The listing builds one solid part. Answer for the finished solid, in the listing's coordinates (mm). A direction names the side the tool comes from. Give positions to 0.01 mm unless a question says otherwise; leave off trailing zeros. Write each loop counter-clockwise with the first axis right and the second up, starting at its lowest first coordinate (ties: lowest second). Pieces come first, ordered by that corner, then holes. Notation, with made-up numbers: (2, -36) -> (36, -36) arc R21 cw to (36, -20) -> close; hole circle Ø6 at (9, 80.5). An arc over 180 degrees is marked (long way). Put each result on its own line as item: value. Start each with the question number.
1) A cutting plane is placed at B-B (y = 9.5). Write down the section's boundary in (x, z).
2) Find the intervals of material crossed by line 1 along X through (y, z) = (-8.75, 1.85); line 2 along X through (y, z) = (-0.75, 2.45); line 3 along Y through (x, z) = (12.5, 2.5), in increasing order. Write a range as from..to.
3) For a pull along X with two mould halves and no side action, classify faces 6 (the cylindrical face through (25.7, 0.5, 1.5)), 7 (the flat face through (20, -13.25, 1)), 8 (the flat face through (-36.5, 9, 1)) as released by +X, released by -X, zero draft, split by the parting line, or undercut.
4) Flat-ended cylindrical pins translate along their axes: pin 1 Ø2 at (y, z) = (-7.5, 1.5) entering from +X; pin 2 Ø0.9 at (y, z) = (9, 1.5) entering from -X; pin 3 Ø1.5 at (x, y) = (24, -1) entering from +Z; pin 4 Ø0.7 at (x, z) = (-38, 1.5) entering from -Y. Find the tip coordinate at first contact, or state that the pin passes through.
5) A cutting plane is placed at A-A (x = 14). Write down the section's boundary in (y, z).
6) For faces 1 (the cylindrical face through (-18.07, -10.7, 1.52)), 2 (the flat face through (36.5, -5, 1)), 3 (the flat face through (-39, 2.25, 1)), 4 (the flat face through (38, 6.25, 1)), 5 (the cylindrical face through (38.59, 2.71, 3.52)), determine the directions among +Z, -Z, +X, -X, +Y, -Y from which every point of the face is accessible in a straight line to the end or side of a thin tool.
7) A cutting plane is placed at C-C (y = -2). Give the number of separate pieces and of enclosed holes in the cut face, then the cut area to 3 significant figures.
from build123d import *

# Parameters (mm, degrees)
F0_W     = 4
F0_H     = 4
F1_DEPTH = 4
F2_R     = 1.6
F3_R     = 1.5
F4_R     = 1


with BuildPart() as f1:
    # F0 (on Top) → F1 (new body)
    with BuildSketch(Plane.XY):
        with BuildLine():
            Line((36.5, 6.25), (36.5, 13.25))
            Line((36.5, 13.25), (-36.5, 13.25))
            Line((-36.5, 13.25), (-36.5, 6.25))
            Line((-36.5, 6.25), (-36.5, 2.25))
            Line((-36.5, 2.25), (-36.5, -13.25))
            Line((-36.5, -13.25), (-29.5, -13.25))
            Line((-29.5, -13.25), (-29.5, -3.25))
            ThreePointArc((-29.5, -3.25), (-25.75, 0.5), (-22, -3.25))
            Line((-22, -3.25), (-22, -13.25))
            Line((-22, -13.25), (-18.5, -13.25))
            Line((-18.5, -13.25), (-18.5, -10.25))
            Line((-18.5, -10.25), (18.5, -10.25))
            Line((18.5, -10.25), (18.5, -13.25))
            Line((18.5, -13.25), (22, -13.25))
            Line((22, -13.25), (22, -3.25))
            ThreePointArc((22, -3.25), (25.75, 0.5), (29.5, -3.25))
            Line((29.5, -3.25), (29.5, -13.25))
            Line((29.5, -13.25), (36.5, -13.25))
            Line((36.5, -13.25), (36.5, 2.25))
            Line((36.5, 2.25), (36.5, 6.25))
        make_face()
        with Locations((-38.5, 4.25)):
            Rectangle(F0_W, F0_H)
        with Locations((38.5, 4.25)):
            Rectangle(F0_W, F0_H)
    extrude(amount=F1_DEPTH)

    # F2
    f2_edges = [f1.edges().sort_by_distance(p)[0] for p in [
        (38.5, 6.25, 4),
        (38.5, 2.25, 4),
        (-38.5, 2.25, 4),
        (-38.5, 6.25, 4),
    ]]
    fillet(f2_edges, radius=F2_R)

    # F3
    f3_edges = [f1.edges().sort_by_distance(p)[0] for p in [
        (-18.5, -10.25, 2),
        (18.5, -10.25, 2),
    ]]
    fillet(f3_edges, radius=F3_R)

    # F4
    f4_edges = [f1.edges().sort_by_distance(p)[0] for p in [
        (-36.5, -13.25, 2),
        (-29.5, -13.25, 2),
        (-22, -13.25, 2),
        (-18.5, -13.25, 2),
        (18.5, -13.25, 2),
        (22, -13.25, 2),
        (29.5, -13.25, 2),
        (36.5, -13.25, 2),
        (-36.5, 13.25, 2),
        (36.5, 13.25, 2),
        (36.5, -5.5, 4),
        (0, 13.25, 4),
        (36.5, 9.75, 4),
        (-36.5, 9.75, 4),
        (-36.5, -5.5, 4),
        (-22, -8.25, 4),
        (22, -8.25, 4),
        (0, -10.25, 4),
        (-33, -13.25, 4),
        (33, -13.25, 4),
        (20.25, -13.25, 4),
        (-20.25, -13.25, 4),
    ]]
    fillet(f4_edges, radius=F4_R)


solid = f1.part
Reply:
1. outline: (-36.5, 0) -> (36.5, 0) -> (36.5, 3) arc R1 ccw to (35.5, 4) -> (-35.5, 4) arc R1 ccw to (-36.5, 3) -> close
2. line 1: x = -36.5..-29.5, -22..22, 29.5..36.5
2. line 2: x = -36.5..-28.55, -22.95..22.95, 28.55..36.5
2. line 3: y = -10.25..13.25
3. face 6: undercut
3. face 7: zero draft
3. face 8: released by -X
4. pin 1: stops at x = 36.5
4. pin 2: stops at x = -36.5
4. pin 3: passes through
4. pin 4: stops at y = 2.25
5. outline: (-10.25, 0) -> (13.25, 0) -> (13.25, 3) arc R1 ccw to (12.25, 4) -> (-9.25, 4) arc R1 ccw to (-10.25, 3) -> close
6. face 1: +Z, -Z, -Y
6. face 2: +Z, -Z, +X, -Y
6. face 3: +Z, -Z, -X, -Y
6. face 4: +Z, -Z, +X, +Y
6. face 5: +Z, +X, -Y
7. separate pieces: 3
7. enclosed holes: 0
7. area: 234 mm2
